For this review, take the finished solid that the model builds, in its own axes (mm). A direction names the side the tool comes from. Round coordinates to 2 decimals unless told otherwise and drop trailing zeros. Loops run counter-clockwise (first coordinate to the right, second up) from the corner with the lowest first, then second, coordinate; pieces in that order, holes last. Notation, with made-up numbers: (58, 67) -> (85, 67) arc R26 cw to (85, 103) -> close; hole circle Ø2 at (41.25, 81.25). An arc over 180 degrees is marked (long way). Write each question's results on one line, items separated by ' | '.
```python
from build123d import *

# Parameters (mm, degrees)
SKETCH1_R           = 33.02
BOSS_EXTRUDE1_DEPTH = 2.54
SKETCH2_R           = 3.175
BOSS_EXTRUDE2_DEPTH = 2.54
CIRPATTERN1_COUNT   = 3
SKETCH3_W           = 2.54
SKETCH3_H           = 1.27
SKETCH3_R           = 0.5715
BOSS_EXTRUDE3_DEPTH = 2.54
CIRPATTERN8_COUNT   = 6
SKETCH4_R           = 1.036302298
BOSS_EXTRUDE4_DEPTH = 2.54
SKETCH5_R           = 1.269883707
SKETCH5_R_2         = 1.184340282
BOSS_EXTRUDE5_DEPTH = 2.54
CIRPATTERN9_COUNT   = 3


with BuildPart() as part:
    # Sketch1 → Boss-Extrude1 (new body)
    with BuildSketch(Plane.XY):
        Circle(SKETCH1_R)
    extrude(amount=BOSS_EXTRUDE1_DEPTH)

    # Sketch2 → Boss-Extrude2 (add)
    with BuildSketch(Plane.XY.offset(2.54)):
        with Locations((14.605, 25.296602045)):
            Circle(SKETCH2_R)
    boss_extrude2 = extrude(amount=BOSS_EXTRUDE2_DEPTH)

    # CirPattern1: Boss-Extrude2 ×3 about axis
    cirpattern1_axis = Axis((0, 0, 0), (0, 0, 1))
    for i in range(1, CIRPATTERN1_COUNT):
        add(boss_extrude2.rotate(cirpattern1_axis, i * 360 / CIRPATTERN1_COUNT))

    # Sketch3 → Boss-Extrude3 (add)
    with BuildSketch(Plane.XY.offset(2.54)):
        with Locations((0, -27.94)):
            Rectangle(SKETCH3_W, SKETCH3_H)
        with Locations((0, -27.94)):
            Circle(SKETCH3_R, mode=Mode.SUBTRACT)
        with Locations((0, -30.861)):
            Rectangle(SKETCH3_W, SKETCH3_H)
        with Locations((0, -30.861)):
            Circle(SKETCH3_R, mode=Mode.SUBTRACT)
    boss_extrude3 = extrude(amount=BOSS_EXTRUDE3_DEPTH)

    # CirPattern8: Boss-Extrude3 ×6 about axis
    cirpattern8_axis = Axis((0, 0, 0), (0, 0, 1))
    for i in range(1, CIRPATTERN8_COUNT):
        add(boss_extrude3.rotate(cirpattern8_axis, i * 360 / CIRPATTERN8_COUNT))

    # Sketch4 → Boss-Extrude4 (add)
    with BuildSketch(Plane.XY.offset(2.54)):
        with Locations((-3.2512, 21.2979)):
            Circle(SKETCH4_R)
        with Locations((-3.2512, -16.8021)):
            Circle(SKETCH4_R)
        with Locations((3.2512, 21.2979)):
            Circle(SKETCH4_R)
        with Locations((3.2512, 16.8021)):
            Circle(SKETCH4_R)
        with Locations((-3.2512, 16.8021)):
            Circle(SKETCH4_R)
        with Locations((3.2512, -16.8021)):
            Circle(SKETCH4_R)
        with Locations((3.2512, -21.2979)):
            Circle(SKETCH4_R)
        with Locations((-3.2512, -21.2979)):
            Circle(SKETCH4_R)
    extrude(amount=BOSS_EXTRUDE4_DEPTH)

    # Sketch5 → Boss-Extrude5 (add)
    with BuildSketch(Plane.XY.offset(2.54)):
        with Locations((15.24, 0)):
            Circle(SKETCH5_R)
        with Locations((19.05, 0)):
            Circle(SKETCH5_R_2)
    boss_extrude5 = extrude(amount=BOSS_EXTRUDE5_DEPTH)

    # CirPattern9: Boss-Extrude5 ×3 about axis
    cirpattern9_axis = Axis((0, 0, 0), (0, 0, 1))
    for i in range(1, CIRPATTERN9_COUNT):
        add(boss_extrude5.rotate(cirpattern9_axis, i * 360 / CIRPATTERN9_COUNT))


solid = part.part
```
1. To check wall thickness, follow probe 1 along Y at (x, z) = (-1, 2.7) (3 decimals); probe 2 along X at (y, z) = (-13.97, 3.65); probe 3 along Z at (x, y) = (11, 8.5). State the ranges of each line that lie inside material, in increasing order.
Values found:
probe 1: y = -31.496 to -30.226, -28.575 to -27.305, 27.305 to 28.575, 30.226 to 31.496 | probe 2: x = -24.93 to -24.77, -23.63 to -23.46, -8.63 to -6.61, 23.46 to 23.63, 24.77 to 24.93 | probe 3: z = 0 to 2.54
2. Tool access review of faces 4 (the face through (-2.26, 17.11, 3.79)), 5 (the face through (3, 21, 5.08)): name each direction out of +Z, -Z, +X, -X, +Y, -Y from which nothing blocks a thin tool from reaching the whole face with its end or side.
Values found:
face 4: +Z | face 5: +Z, +X, -X, +Y, -Y
3. Consider section D-D (x = -29.21). State the section outline as (y, z) points (3 decimals), plus the area to 3 significant figures.
Values found:
outline: (-15.398, 0) -> (15.398, 0) -> (15.398, 2.54) -> (3.175, 2.54) -> (3.175, 5.08) -> (-3.175, 5.08) -> (-3.175, 2.54) -> (-15.398, 2.54) -> close | area: 94.4 mm2
4. Consider section A-A (x = -3). State the section outline as (y, z) points.
Values found:
outline: (-32.88, 0) -> (32.88, 0) -> (32.88, 2.54) -> (22.3, 2.54) -> (22.3, 5.08) -> (20.29, 5.08) -> (20.29, 2.54) -> (17.81, 2.54) -> (17.81, 5.08) -> (15.8, 5.08) -> (15.8, 2.54) -> (-15.8, 2.54) -> (-15.8, 5.08) -> (-17.81, 5.08) -> (-17.81, 2.54) -> (-20.29, 2.54) -> (-20.29, 5.08) -> (-22.3, 5.08) -> (-22.3, 2.54) -> (-32.88, 2.54) -> close
5. Consider section B-B (z = 3.7). Give the number of separate pieces and of enclosed holes in the cut face, plus the area to 3 significant figures.
Values found:
separate pieces: 29 | enclosed holes: 12 | area: 177 mm2
6. For pin 1 (0.9 mm diameter, centred on x = -26.73, y = 15.43, fed in from +Z); pin 2 (1.3 mm diameter, centred on x = -24.2, y = -13.97, fed in from +Z); pin 3 (1.4 mm diameter, centred on y = 28, z = 4.5, fed in from +X); pin 4 (0.6 mm diameter, centred on y = -28, z = 4, fed in from -X), all flat-tipped, find the tip position at first contact; note any pin that passes through.
Values found:
pin 1: stops at z = 2.54 | pin 2: stops at z = 5.08 | pin 3: stops at x = 17.07 | pin 4: stops at x = -1.27
7. Draft analysis for pull direction X (two halves, no side actions). For faces 1 (the face through (-3.48, -22.31, 3.79)), 2 (the face through (31.5, 9.9, 1.3)), 3 (the face through (-10, -16, 5.08)), state which applies: released by +X, released by -X, zero draft, split by the parting line, or undercut.
Values found:
face 1: undercut | face 2: split by the parting line | face 3: zero draft
8. Consider section C-C (x = 19.05). State the section outline as (y, z) points.
Values found:
outline: (-26.97, 0) -> (26.97, 0) -> (26.97, 2.54) -> (1.18, 2.54) -> (1.18, 5.08) -> (-1.18, 5.08) -> (-1.18, 2.54) -> (-26.97, 2.54) -> close
